Design review of the part built by this model. Coordinates are the model's own, in mm. Give positions to 0.01 mm unless a question says otherwise; leave off trailing zeros. Order: outer loops, then holes, each group sorted by start corner. A loop starts at its lowest first (then second) coordinate and runs counter-clockwise, first axis right, second up.
```python
from build123d import *

# Parameters (mm, degrees)
SKETCH1_W             = 30
SKETCH1_H             = 30
BOSS_EXTRUDE1_DEPTH   = 10
SKETCH2_R             = 5
CUT_EXTRUDE1_DEPTH    = 44.588989435
F_3_0MM_DOWEL_HOLE1_D = 3


with BuildPart() as part:
    # Sketch1 → Boss-Extrude1 (new body)
    with BuildSketch(Plane(origin=(0, 0, 0), x_dir=(1, 0, 0), z_dir=(0, 1, 0))):
        with Locations((15, 15)):
            Rectangle(SKETCH1_W, SKETCH1_H)
    extrude(amount=BOSS_EXTRUDE1_DEPTH)

    # Sketch2 → Cut-Extrude1 (cut, through all)
    with BuildSketch(Plane(origin=(0, 10, 0), x_dir=(1, 0, 0), z_dir=(0, 1, 0))):
        with Locations(Location((15, 15, 0), (0, 0, 270))):
            Circle(SKETCH2_R)
    extrude(amount=-CUT_EXTRUDE1_DEPTH, mode=Mode.SUBTRACT)

    # Ø3.0mm Dowel Hole1 (through all)
    with Locations(Plane(origin=(0, 10, 0), x_dir=(1, 0, 0), z_dir=(0, 1, 0))):
        with Locations((5, 15), (25, 15)):
            Hole(F_3_0MM_DOWEL_HOLE1_D / 2)


solid = part.part
```
1. Take a section at C-C (z = -15.5). State the section outline as (x, y) points, then the cut area to 3 significant figures.
Recorded:
outline: (0, 0) - (3.59, 0) - (3.59, 10) - (0, 10) - close; (6.41, 0) - (10.03, 0) - (10.03, 10) - (6.41, 10) - close; (19.97, 0) - (23.59, 0) - (23.59, 10) - (19.97, 10) - close; (26.41, 0) - (30, 0) - (30, 10) - (26.41, 10) - close
area: 144 mm2
2. Take a section at B-B (y = 8.75). State the section outline as (x, z) points, then the cut area to 3 significant figures.
Recorded:
outline: (0, -30) - (30, -30) - (30, 0) - (0, 0) - close; hole circle Ø3 at (5, -15); hole circle Ø10 at (15, -15); hole circle Ø3 at (25, -15)
area: 807 mm2
3. For pin 1 (8 mm diameter, centred on x = 15, z = -15, fed in from +Y), flat-tipped, find the tip position at first contact; note if it passes through.
Recorded:
pin 1: passes through
4. Take a section at D-D (x = 18). State the section outline as (y, z) points, then the cut area to 3 significant figures.
Recorded:
outline: (0, -30) - (10, -30) - (10, -19) - (0, -19) - close; (0, -11) - (10, -11) - (10, 0) - (0, 0) - close
area: 220 mm2
5. For line 1 along X through (y, z) = (6.75, -15); line 2 along Z through (x, y) = (5, 4); line 3 along Z through (x, y) = (4, 1.25), list the stretches that pass through material, from the lowest coordinate up.
Recorded:
line 1: x = 0 to 3.5, 6.5 to 10, 20 to 23.5, 26.5 to 30
line 2: z = -30 to -16.5, -13.5 to 0
line 3: z = -30 to -16.12, -13.88 to 0
6. Take a section at A-A (x = 15). State the section outline as (y, z) points.
Recorded:
outline: (0, -30) - (10, -30) - (10, -20) - (0, -20) - close; (0, -10) - (10, -10) - (10, 0) - (0, 0) - close
